```python
from build123d import *

# Parameters (mm, degrees)
F1_DEPTH = 19.05
F2_R     = 12.7
F4_DEPTH = 25.4


with BuildPart() as f1:
    # F0 (on Front) → F1 (new body, symmetric)
    with BuildSketch(Plane.XZ):
        Polygon((-25.4, 12.7), (-63.5, 12.7), (-63.5, -12.7), (63.5, -12.7), (63.5, 12.7), (25.4, 12.7), (0, 12.7), align=None)
        Polygon((-25.4, 63.5), (-25.4, 12.7), (0, 12.7), (25.4, 12.7), (25.4, 63.5), (0, 63.5), align=None)
        with BuildLine():
            ThreePointArc((12.7, 38.1), (-8.980256, 29.119744), (0, 50.8))
            ThreePointArc((0, 50.8), (8.980256, 47.080256), (12.7, 38.1))
        make_face(mode=Mode.SUBTRACT)
    extrude(amount=F1_DEPTH, both=True)

    # F2
    f2_edges = [f1.edges().sort_by_distance(p)[0] for p in [
        (-25.4, 0, 63.5),
        (25.4, 0, 63.5),
    ]]
    fillet(f2_edges, radius=F2_R)

    # F3 (on face) → F4 (cut, symmetric)
    with BuildSketch(Plane.XY.offset(12.7)):
        with BuildLine():
            ThreePointArc((38.1, 0), (44.45, -6.35), (50.8, 0))
            ThreePointArc((50.8, 0), (44.45, 6.35), (38.1, 0))
        make_face()
        with BuildLine():
            ThreePointArc((-50.8, 0), (-44.45, -6.35), (-38.1, 0))
            ThreePointArc((-38.1, 0), (-44.45, 6.35), (-50.8, 0))
        make_face()
    extrude(amount=F4_DEPTH, both=True, mode=Mode.SUBTRACT)


solid = f1.part
```
Design review of the part built by this model. Coordinates are the model's own, in mm. A direction names the side the tool comes from. Coordinates: 2 decimals unless noted, no trailing zeros. Loops run counter-clockwise (first coordinate to the right, second up) from the corner with the lowest first, then second, coordinate; pieces in that order, holes last. Notation, with made-up numbers: (45.25, 70) -> (92.25, 70) arc R17 cw to (92.25, 93) -> close; hole circle Ø10 at (-34, -8). An arc over 180 degrees is marked (long way). Answer as a JSON object with one key per item and string values.
Q1. The part is to be moulded in two halves that separate along X. For faces 4 (the cylindrical face through (50.507, 1.907, 0.178)), 5 (the flat face through (-63.5, 0, 0)), 6 (the flat face through (-40, -5, 12.7)), say which applies: +X half, -X half, draft (parallel to the pull), parting line (faces both ways), or undercut.
Answer block:
{"face 4": "undercut", "face 5": "-X half", "face 6": "draft"}
Q2. Take a section at D-D on z = 7.5. Give the boundary of the cut face in (x, y), plus the area to 3 significant figures.
Answer block:
{"outline": "(-63.5, -19.05) -> (63.5, -19.05) -> (63.5, 19.05) -> (-63.5, 19.05) -> close; hole circle Ø12.7 at (-44.45, 0); hole circle Ø12.7 at (44.45, 0)", "area": "4,590 mm^2"}
Q3. Tool access review of faces 1 (the flat face through (0, 0, 63.5)), 2 (the flat face through (49, -5, 12.7)), 3 (the flat face through (-25.4, 0, 32)): name each direction out of +Z, -Z, +X, -X, +Y, -Y from which nothing blocks a thin tool from reaching the whole face with its end or side.
Answer block:
{"face 1": "+Z, +X, -X, +Y, -Y", "face 2": "+Z, +X, +Y, -Y", "face 3": "+Z, -X, +Y, -Y"}
Q4. Take a section at A-A on y = 0. Give the boundary of the cut face in (x, z), plus the area to 3 significant figures.
Answer block:
{"outline": "(-63.5, -12.7) -> (-50.8, -12.7) -> (-50.8, 12.7) -> (-63.5, 12.7) -> close; (-38.1, -12.7) -> (38.1, -12.7) -> (38.1, 12.7) -> (25.4, 12.7) -> (25.4, 50.8) arc R12.7 ccw to (12.7, 63.5) -> (-12.7, 63.5) arc R12.7 ccw to (-25.4, 50.8) -> (-25.4, 12.7) -> (-38.1, 12.7) -> close; (50.8, -12.7) -> (63.5, -12.7) -> (63.5, 12.7) -> (50.8, 12.7) -> close; hole circle Ø25.4 at (0, 38.1)", "area": "4,590 mm^2"}
Q5. To check wall thickness, follow L1, parallel to X at y = -4, z = 38.1; L2, parallel to Y at x = -44.45, z = -7.5; L3, parallel to Z at x = -13, y = 12.5. State the ranges of each line that lie inside material, in increasing order.
Answer block:
{"L1": "x = -25.4 to -12.7, 12.7 to 25.4", "L2": "y = -19.05 to -6.35, 6.35 to 19.05", "L3": "z = -12.7 to 63.5"}
Q6. Take a section at B-B on x = 44.45. Give the boundary of the cut face in (y, z).
Answer block:
{"outline": "(-19.05, -12.7) -> (-6.35, -12.7) -> (-6.35, 12.7) -> (-19.05, 12.7) -> close; (6.35, -12.7) -> (19.05, -12.7) -> (19.05, 12.7) -> (6.35, 12.7) -> close"}
Q7. Clearance check with flat-ended pins moving along their axes: pin 1 Ø4 at (y, z) = (9, 33.5) entering from +X; pin 2 Ø16.5 at (x, y) = (-44.45, 0) entering from +Z; pin 3 Ø11.5 at (y, z) = (-8.5, 34.5) entering from -X. State where each tip first meets the part, or that it passes through.
Answer block:
{"pin 1": "stops at x = 25.4", "pin 2": "stops at z = 12.7", "pin 3": "stops at x = -25.4"}
Q8. Take a section at C-C on y = -14. Give the boundary of the cut face in (x, z), plus the area to 3 significant figures.
Answer block:
{"outline": "(-63.5, -12.7) -> (63.5, -12.7) -> (63.5, 12.7) -> (25.4, 12.7) -> (25.4, 50.8) arc R12.7 ccw to (12.7, 63.5) -> (-12.7, 63.5) arc R12.7 ccw to (-25.4, 50.8) -> (-25.4, 12.7) -> (-63.5, 12.7) -> close; hole circle Ø25.4 at (0, 38.1)", "area": "5,230 mm^2"}
